The listing builds one solid part. Answer for the finished solid, in the listing's coordinates (mm). A direction names the side the tool comes from. Give positions to 0.01 mm unless a question says otherwise; leave off trailing zeros. Write each loop counter-clockwise with the first axis right and the second up, starting at its lowest first coordinate (ties: lowest second). Pieces come first, ordered by that corner, then holes. Notation, with made-up numbers: (32, 50) - (46, 50) arc R9 cw to (46, 57) - close; hole circle Ø3 at (-29, 1.25). An arc over 180 degrees is marked (long way). Write each question's results on one line, items separated by ' | '. Start each with the question number.
Q1. For a pull along Z with two mould halves and no side action, classify faces 1 (the face through (32.737, -2.465, 7.676)), 2 (the face through (21, -7, 0)), 3 (the face through (42, -6, 7)), 4 (the face through (17, -6.9, 5.5)) as pulls with the +Z half, pulls with the -Z half, needs draft (parallel to the pull), parting line crosses it, or undercut.
Q2. Section D-D (y = -7) is taken. Determine the outline of the cut face in (x, z), plus the area to 3 significant figures.
Q3. Section B-B (z = 7) is taken. Determine the outline of the cut face in (x, y).
Q4. Find the intervals of material crossed by probe 1 along X at (y, z) = (-7.75, 4); probe 2 along Z at (x, y) = (32, -3.6); probe 3 along X at (y, z) = (-9, 7.75), in increasing order.
Q5. A flat-ended cylindrical pin translates along its axis: pin 1 Ø1 at (x, z) = (19, 7) entering from +Y. Find the tip coordinate at first contact, or state that the pin passes through.
Q6. Section A-A (x = 15) is taken. Determine the outline of the cut face in (y, z).
Q7. For faces 5 (the face through (21, 0, 7)), 6 (the face through (32, -5, 7)), determine the directions among +Z, -Z, +X, -X, +Y, -Y from which every point of the face is accessible in a straight line to the end or side of a thin tool.
Q8. Section C-C (y = -2) is taken. Determine the outline of the cut face in (x, z), plus the area to 3 significant figures.
```python
from build123d import *

# Parameters (mm, degrees)
F0_W     = 42
F0_H     = 14
F1_DEPTH = 14
F3_DEPTH = 25
F5_DEPTH = 5
F6_R     = 2.5
F7_DEPTH = 25
F8_SIZE  = 3


with BuildPart() as f1:
    # F0 (on Top) → F1 (new body)
    with BuildSketch(Plane.XY):
        with Locations((21, -7)):
            Rectangle(F0_W, F0_H)
    extrude(amount=F1_DEPTH)

    # F2 (on face) → F3 (cut)
    with BuildSketch(Plane.XY.offset(14)):
        with BuildLine():
            ThreePointArc((5, -10.5), (6.06066, -10.06066), (6.5, -9))
            ThreePointArc((6.5, -9), (3.93934, -7.93934), (5, -10.5))
        make_face()
        with BuildLine():
            ThreePointArc((37, -10.5), (38.06066, -10.06066), (38.5, -9))
            ThreePointArc((38.5, -9), (35.93934, -7.93934), (37, -10.5))
        make_face()
    extrude(amount=-F3_DEPTH, mode=Mode.SUBTRACT)

    # F4 (on face) → F5 (cut)
    with BuildSketch(Plane(origin=(0, 0, 0), x_dir=(-1, 0, 0), z_dir=(0, 1, 0))):
        with BuildLine():
            ThreePointArc((-33, 7), (-32, 6), (-31, 7))
            ThreePointArc((-31, 7), (-32, 8), (-33, 7))
        make_face()
    extrude(amount=-F5_DEPTH, mode=Mode.SUBTRACT)

    # F6 (on face) → F7 (cut)
    with BuildSketch(Plane(origin=(0, 0, 0), x_dir=(-1, 0, 0), z_dir=(0, 1, 0))):
        with Locations((-15, 7)):
            Circle(F6_R)
    extrude(amount=-F7_DEPTH, mode=Mode.SUBTRACT)

    # F8
    f8_edges = [f1.edges().sort_by_distance(p)[0] for p in [
        (0, -14, 7),
        (42, -14, 7),
    ]]
    chamfer(f8_edges, length=F8_SIZE)


solid = f1.part
```
Answers below:
1) face 1: undercut | face 2: pulls with the -Z half | face 3: needs draft | face 4: undercut
2) outline: (0, 0) - (42, 0) - (42, 14) - (0, 14) - close; hole circle Ø5 at (15, 7) | area: 568 mm2
3) outline: (0, -11) - (3, -14) - (12.5, -14) - (12.5, 0) - (0, 0) - close; (17.5, -14) - (39, -14) - (42, -11) - (42, 0) - (33, 0) - (33, -5) - (31, -5) - (31, 0) - (17.5, 0) - close; hole circle Ø3 at (5, -9); hole circle Ø3 at (37, -9)
4) probe 1: x = 0 to 4.17, 5.83 to 36.17, 37.83 to 42 | probe 2: z = 0 to 6, 8 to 14 | probe 3: x = 0 to 3.5, 6.5 to 12.62, 17.38 to 35.5, 38.5 to 42
5) pin 1: stops at y = 0
6) outline: (-14, 0) - (0, 0) - (0, 4.5) - (-14, 4.5) - close; (-14, 9.5) - (0, 9.5) - (0, 14) - (-14, 14) - close
7) face 5: +Z, -Z, +X, -X, +Y | face 6: +Y
8) outline: (0, 0) - (42, 0) - (42, 14) - (0, 14) - close; hole circle Ø5 at (15, 7); hole circle Ø2 at (32, 7) | area: 565 mm2
